```python
from build123d import *

# Parameters (mm, degrees)
SKETCH_1_W      = 70
SKETCH_1_H      = 30
EXTRUDE_1_DEPTH = 18
FILLET_1_R      = 6
SKETCH_2_W      = 15
SKETCH_2_H      = 3
SKETCH_2_H_2    = 18
EXTRUDE_2_DEPTH = 12
FILLET_2_R      = 6


with BuildPart() as part:
    # 草图1 → 凸台-拉伸1 (new body)
    with BuildSketch(Plane(origin=(0, 0, 0), x_dir=(1, 0, 0), z_dir=(0, 1, 0))):
        Rectangle(SKETCH_1_W, SKETCH_1_H)
    extrude(amount=EXTRUDE_1_DEPTH)

    # 圆角1
    fillet_1_edges = [part.edges().sort_by_distance(p)[0] for p in [
        (-35, 9, 15),
        (-35, 9, -15),
    ]]
    fillet(fillet_1_edges, radius=FILLET_1_R)

    # 草图2 → 凸台-拉伸2 (add)
    with BuildSketch(Plane.ZY.offset(35)):
        with Locations((0, 19.5)):
            Rectangle(SKETCH_2_W, SKETCH_2_H)
        with Locations((0, 9)):
            Rectangle(SKETCH_2_W, SKETCH_2_H_2)
    extrude(amount=EXTRUDE_2_DEPTH)

    # 圆角2
    # the kernel refuses this fillet: 6 mm, written as the material it adds along each edge
    with BuildSketch(Plane(origin=(-35, 18, 7.5), x_dir=(1, 0, 0), z_dir=(0, 0, -1))) as fillet_2_piece_1:
        with BuildLine():
            CenterArc((5.196152423, -6), FILLET_2_R, 90, 60)
            Line((0, -3), (0, 0))
            Line((0, 0), (5.196152423, 0))
        make_face()
    extrude(amount=15)


solid = part.part
```
Input: part model. Units: mm. Frame: model coordinates. A direction names the side the tool comes from. Round coordinates to 2 decimals unless told otherwise and drop trailing zeros. Write each loop counter-clockwise with the first axis right and the second up, starting at its lowest first coordinate (ties: lowest second). Pieces come first, ordered by that corner, then holes. Notation, with made-up numbers: (26.25, -5.75) -> (34.25, -5.75) arc R13 ccw to (34.25, 18.25) -> close; hole circle Ø7 at (42.25, 49). An arc over 180 degrees is marked (long way). Answer as CSV lines item,"result".
1. Contact query for flat-ended pins moving along their axis: P1, Ø1.6, axis at y = 12.5, z = -8.5, coming from the -X side; P2, Ø1.5, axis at x = -6.5, z = -6, coming from the +Y side; P3, Ø8.5, axis at x = -38, y = 12, coming from the +Z side. Output: stop coordinate, or through.
Geometry says:
P1,"stops at x = -35"
P2,"stops at y = 18"
P3,"stops at z = 12.67"
2. Reachability of faces 1 (the flat face through (-35, 9, -8)), 2 (the flat face through (-35, 9, 8)), 3 (the flat face through (3, 9, -15)) from +Z, -Z, +X, -X, +Y, -Y: full face, straight path, thin tool, end or side. Return the list, or none.
Geometry says:
face 1,"-Z, -X, +Y, -Y"
face 2,"+Z, -X, +Y, -Y"
face 3,"-Z, +X, -X, +Y, -Y"
3. Section C-C (x = -21). Return the cut outline in (y, z), plus the area to 3 significant figures.
Geometry says:
outline,"(0, -15) -> (18, -15) -> (18, 15) -> (0, 15) -> close"
area,"540 mm^2"
4. Section D-D (x = -40). Return the cut outline in (y, z), plus the area to 3 significant figures.
Geometry says:
outline,"(0, -7.5) -> (21, -7.5) -> (21, 7.5) -> (0, 7.5) -> close"
area,"315 mm^2"
5. Section B-B (z = 3.75). Return the cut outline in (x, y).
Geometry says:
outline,"(-47, 0) -> (35, 0) -> (35, 18) -> (-29.8, 18) arc R6 cw to (-35, 21) -> (-47, 21) -> close"
6. Ray query, L1, parallel to Z at x = -36.5, y = 8.5; L2, parallel to Y at x = 5, z = 0; L3, parallel to X at y = 8, z = 9.25. Return the intervals inside material, ascending. Write a range as [from, to].
Geometry says:
L1,"z = [-7.5, 7.5]"
L2,"y = [0, 18]"
L3,"x = [-34.99, 35]"
7. Section A-A (y = 13.5). Return the cut outline in (x, z).
Geometry says:
outline,"(-47, -7.5) -> (-35, -7.5) -> (-35, -9) arc R6 ccw to (-29, -15) -> (35, -15) -> (35, 15) -> (-29, 15) arc R6 ccw to (-35, 9) -> (-35, 7.5) -> (-47, 7.5) -> close"
